from build123d import *

# Parameters (mm, degrees)
F0_W     = 15
F0_H     = 15
F0_R     = 2
F0_R_2   = 4.25
F1_DEPTH = 2
F0_R_3   = 4
F2_DEPTH = 2.65
F0_R_4   = 3.7599999923
F0_R_5   = 3
F3_DEPTH = 7.5
F0_R_6   = 2.15
F4_DEPTH = 3.5
F5_DEPTH = 2.5
F6_SIZE  = 1.5
F0_R_7   = 1.15
F7_DEPTH = 0.5


with BuildPart() as f1:
    # F0 (on Top) → F1 (new body)
    with BuildSketch(Plane.XY):
        Rectangle(F0_W, F0_H)
        with Locations((-5, -5)):
            Circle(F0_R, mode=Mode.SUBTRACT)
        with Locations((5, -5)):
            Circle(F0_R, mode=Mode.SUBTRACT)
        with Locations((-5, 5)):
            Circle(F0_R, mode=Mode.SUBTRACT)
        Circle(F0_R_2, mode=Mode.SUBTRACT)
        with Locations((5, 5)):
            Circle(F0_R, mode=Mode.SUBTRACT)
    extrude(amount=F1_DEPTH)

    # F0 (on Top) → F2 (join)
    with BuildSketch(Plane.XY):
        Circle(F0_R_2)
        Circle(F0_R_3, mode=Mode.SUBTRACT)
    extrude(amount=F2_DEPTH)

    # F0 (on Top) → F3 (join)
    with BuildSketch(Plane.XY):
        Circle(F0_R_3)
        Circle(F0_R_4, mode=Mode.SUBTRACT)
        Circle(F0_R_4)
        Circle(F0_R_5, mode=Mode.SUBTRACT)
    extrude(amount=F3_DEPTH)

    # F0 (on Top) → F4 (join)
    with BuildSketch(Plane.XY):
        Circle(F0_R_4)
        Circle(F0_R_5, mode=Mode.SUBTRACT)
        Circle(F0_R_5)
        Circle(F0_R_6, mode=Mode.SUBTRACT)
    extrude(amount=F4_DEPTH)

    # F0 (on Top) → F5 (cut)
    with BuildSketch(Plane.XY):
        Circle(F0_R_5)
        Circle(F0_R_6, mode=Mode.SUBTRACT)
    extrude(amount=F5_DEPTH, mode=Mode.SUBTRACT)

    # F6
    f6_edges = [f1.edges().sort_by_distance(p)[0] for p in [
        (7.5, -7.5, 1),
        (7.5, 7.5, 1),
        (-7.5, -7.5, 1),
        (-7.5, 7.5, 1),
    ]]
    chamfer(f6_edges, length=F6_SIZE)

    # F0 (on Top) → F7 (join)
    with BuildSketch(Plane.XY):
        with Locations((-5, 5)):
            Circle(F0_R)
        with Locations((-5, 5)):
            Circle(F0_R_7, mode=Mode.SUBTRACT)
        with Locations((5, 5)):
            Circle(F0_R)
        with Locations((5, 5)):
            Circle(F0_R_7, mode=Mode.SUBTRACT)
        with Locations((5, -5)):
            Circle(F0_R)
        with Locations((5, -5)):
            Circle(F0_R_7, mode=Mode.SUBTRACT)
        with Locations((-5, -5)):
            Circle(F0_R)
        with Locations((-5, -5)):
            Circle(F0_R_7, mode=Mode.SUBTRACT)
    extrude(amount=F7_DEPTH)


solid = f1.part
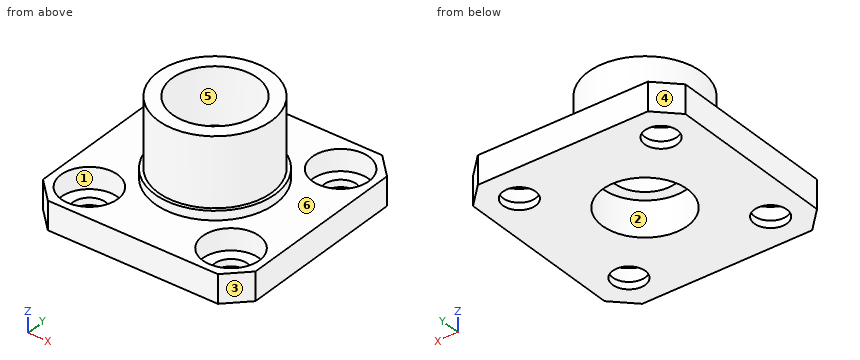
Geometry check sheet. Reference: the model listing, model coordinates, mm. Face numbers are marked on the shaded views. A direction names the side the tool comes from. Give positions to 0.01 mm unless a question says otherwise; leave off trailing zeros. Write each loop counter-clockwise with the first axis right and the second up, starting at its lowest first coordinate (ties: lowest second). Pieces come first, ordered by that corner, then holes. Notation, with made-up numbers: M 6.5,-5.75 L 18.5,-5.75 A11 cw 18.5,1.25 Z; hole C 54,25.25 d2. An arc over 180 degrees is marked long. Answer as CSV lines item,"result". Start each with the question number.
Q1. Section check B-B, the plane y = 0. Record the cut outline in (x, z), then the cut area to 3 significant figures.
Q2. Release check for a two-part mould opening along X. For the marked faces 4, 5 and 6 record: pulls with the +X half, pulls with the -X half, needs draft (parallel to the pull), parting line crosses it, or undercut.
Q3. Material ranges on L1, parallel to Y at x = -5, z = 1.2; L2, parallel to Y at x = 0, z = 1.65; L3, parallel to Z at x = -3.5, y = 3, recorded low to high.
Q4. Tool access check on the marked faces 1, 2 and 3. Record the directions out of +Z, -Z, +X, -X, +Y, -Y that give a thin tool (end or side, any length) a straight path to the whole face; none if there is none.
Q5. Go/stop test with flat-tipped pins: pin 1 (4.5 mm diameter, centred on x = -4.5, y = 6, fed in from +Z); pin 2 (3.5 mm diameter, centred on x = 5, y = 5, fed in from +Z); pin 3 (4 mm diameter, centred on y = -3.5, z = 5, fed in from -X); pin 4 (1.8 mm diameter, centred on x = -5, y = 5, fed in from +Z). Record where each tip stops, or that it passes through.
Q6. Section check A-A, the plane x = 5. Record the cut outline in (y, z).
Q7. Section check D-D, the plane y = 4.5. Record the cut outline in (x, z).
Geometry says:
1,outline,"M -7.5,0 L -3,0 L -3,2.5 L -2.15,2.5 L -2.15,3.5 L -3,3.5 L -3,7.5 L -4,7.5 L -4,2.65 L -4.25,2.65 L -4.25,2 L -7.5,2 Z; M 2.15,2.5 L 3,2.5 L 3,0 L 7.5,0 L 7.5,2 L 4.25,2 L 4.25,2.65 L 4,2.65 L 4,7.5 L 3,7.5 L 3,3.5 L 2.15,3.5 Z"
1,area,"31.0 mm^2"
2,face 4,"pulls with the -X half"
2,face 5,"undercut"
2,face 6,"needs draft"
3,L1,"-7.5 to -7, -3 to 3, 7 to 7.5"
3,L2,"-7.5 to -3, 3 to 7.5"
3,L3,"0 to 2"
4,face 1,"+Z"
4,face 2,"-Z"
4,face 3,"+Z, -Z, +X, -Y"
5,pin 1,"z = 2"
5,pin 2,"z = 0.5"
5,pin 3,"x = -3.71"
5,pin 4,"through"
6,outline,"M -7.5,0 L -6.15,0 L -6.15,0.5 L -7,0.5 L -7,2 L -7.5,2 Z; M -3.85,0 L 3.85,0 L 3.85,0.5 L 3,0.5 L 3,2 L -3,2 L -3,0.5 L -3.85,0.5 Z; M 6.15,0 L 7.5,0 L 7.5,2 L 7,2 L 7,0.5 L 6.15,0.5 Z"
7,outline,"M -7.5,0 L -6.04,0 L -6.04,0.5 L -6.94,0.5 L -6.94,2 L -7.5,2 Z; M -3.96,0 L 3.96,0 L 3.96,0.5 L 3.06,0.5 L 3.06,2 L -3.06,2 L -3.06,0.5 L -3.96,0.5 Z; M 6.04,0 L 7.5,0 L 7.5,2 L 6.94,2 L 6.94,0.5 L 6.04,0.5 Z"
